Work out the finished part from the listing and answer in its coordinate system (mm). Face numbers are marked on the shaded views. A direction names the side the tool comes from. Give positions to 0.01 mm unless a question says otherwise; leave off trailing zeros. Loops run counter-clockwise (first coordinate to the right, second up) from the corner with the lowest first, then second, coordinate; pieces in that order, holes last. Notation, with made-up numbers: (86.5, 22) - (104.5, 22) arc R22 cw to (104.5, 36) - close; hole circle Ø1 at (61.25, -15.75). An arc over 180 degrees is marked (long way). One line per item, written item: value.
Autodesk Inventor part; units mm, degrees
ref_plane "Work Plane1" through (29, 0, 0) normal (0, -1, 0) x (1, 0, 0)
ref_plane "YZ Plane" through (0, 0, 0) normal (1, 0, 0) x (0, 1, 0)
ref_plane "XZ Plane" through (0, 0, 0) normal (0, 1, 0) x (-1, 0, 0)
sketch "Sketch1" plane through (0, 0, 0) normal (0, 0, 1) x (1, 0, 0)
  line L0 (-0.8667, 0) -> (5, 0)
  line L1 (5, 0) -> (5, 1.5)
  line L2 (5, 1.5) -> (1.25, 1.5)
  line L3 (1.25, 1.5) -> (0.9432, 1.5)
  line L4 (0.9432, 1.5) -> (0, 1.5)
  line L5 (0, 1.5) -> (0, 2.75)
  line L6 (0, 2.75) -> (-3, 2.75)
  line L7 (-3, 2.75) -> (-3, 1.4434)
  line L8 (-3, 1.4434) -> (-1.7, 1.4434)
  line L9 (-1.7, 1.4434) -> (-0.8667, 0)
  line L10 (-4.6, 0) -> (6.6, 0)
  line L11 (0, -0.55) -> (0, 3.3)
  line L12 (1.25, 1.5) -> (0, 1.5) construction
  dimension "d1" = 3.75
  dimension "d2" = 0.3068
  dimension "d3" = 3
  dimension "d4" = 1.3
  dimension "d5" = 60
  dimension "d6" = 3
  dimension "d7" = 3
  dimension "d8" = 2.8868
  dimension "d9" = 5.5
  dimension "d26" = 5
revolve "Body" add sketch "Sketch1" angle 360 about axis through (-0.8667, 0, 0) along (1, 0, 0)
sketch "Sketch2" plane through (-3, 0, 0) normal (-1, 0, 0) x (0, 0, 1)
  circle A0 centre (0, 0) radius 1.4434
  line L0 (0, -3.85) -> (0, 3.85)
  line L1 (-3.85, 0) -> (3.85, 0)
  line L2 (1.4434, 0) -> (0.7217, -1.25)
  line L3 (0.7217, -1.25) -> (-0.7217, -1.25)
  line L4 (-0.7217, -1.25) -> (-1.4434, 0)
  line L5 (-1.4434, 0) -> (-0.7217, 1.25)
  line L6 (-0.7217, 1.25) -> (0.7217, 1.25)
  line L7 (0.7217, 1.25) -> (1.4434, 0)
extrude "Slot" add sketch "Sketch2" against normal up to next contours L7 A0 | A0 L2 | L6 L0 A0 | A0 L0 L3 | L0 L6 A0 | A0 L3 L0 | L4 A0 | A0 L5
fillet "Fillet1" radius 0.3 1 edges at (-3, -2.75, 0)
thread "Thread"
chamfer "Chamfer1" distance 0.3067 distance2 0.3067 1 edges at (5, -1.5, 0) measured on face at (5, -0.2617, -0.7882)
ref_plane "Work Plane1" through (29, 0, 0) normal (0, -1, 0) x (1, 0, 0)
fillet "Fillet2" radius 0.1 1 edges at (0, -1.5, 0)
sketch "Sketch4" plane through (5, 0, 0) normal (1, 0, 0) x (0, 0, -1)
  circle A0 centre (0, 0) radius 2.75
  circle A1 centre (0, 0) radius 1.6
  point P0 (0, 0)
extrude "Extrusion3" cut sketch "Sketch4" against normal blind 1 contours A1
chamfer "Chamfer3" distance 0.5 angle 45 1 edges at (4, -1.5, 0)
equation "\"d1\" = GEL"
equation "\"d3\" = KOH"
equation "\"d4\" = INTI"
equation "\"d6\" = GD"
equation "\"d7\" = BDM"
equation "\"d8\" = 1.1547 * SW"
equation "\"d9\" = KOD"
equation "\"d26\" = NLG"
equation "\"d30\" = R"
equation "\"d17\" = RR"
equation "\"d13\" = GEL"
equation "\"d15\" = -0.5 * SPD + 0.5 * GD"
equation "\"d16\" = GUL"
equation "\"GD\" = 3"
equation "\"NLG\" = 5"
equation "\"GEL\" = 3.75"
equation "\"KOD\" = 5.5"
equation "\"KOH\" = 3"
equation "\"INTI\" = 1.3"
equation "\"GAL\" = 0.61345 * PTC"
equation "\"GUL\" = 0.61345 * PTC"
equation "\"BDM\" = NND"
equation "\"SW\" = 2.5"
equation "\"RR\" = 0.3"
equation "\"SPD\" = NND - 1.2269 * PTC"
equation "\"R\" = 0.1"
equation "\"TOA\" = 30deg"
equation "\"GD1\" = THREADDIA - 1.2269 * PTC"
equation "\"THREADDIA\" = 3"
equation "\"FAWI\" = 45deg"
equation "\"PTC\" = 0.5"
equation "\"NND\" = 3"
equation "\"E0\" = 1.155 * SW"
properties part number "ISO 4762 - M3 x 4" material "Stainless Steel, 440C"
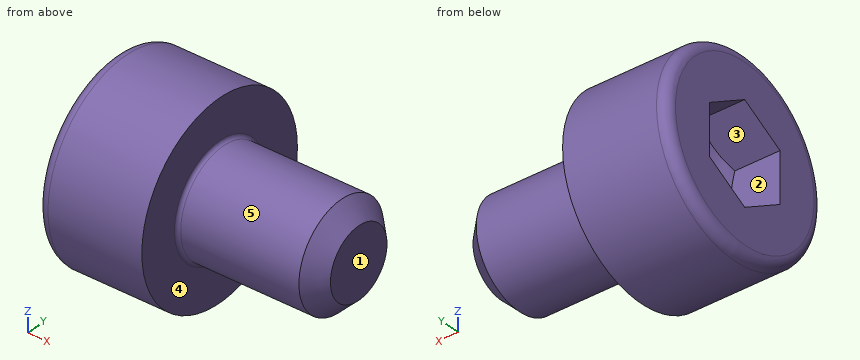
1. The mould has two halves that part along Y. Classify the marked faces 3, 4 and 5: released by +Y, released by -Y, zero draft, split by the parting line, or undercut.
Output:
face 3: undercut
face 4: zero draft
face 5: split by the parting line
2. For the marked faces 1 and 2, determine the directions among +Z, -Z, +X, -X, +Y, -Y from which every point of the face is accessible in a straight line to the end or side of a thin tool.
Output:
face 1: +Z, -Z, +X, +Y, -Y
face 2: -X
3. Section A-A (x = 1.75) is taken. Write down the section's boundary in (y, z), and give its area (3 significant figures).
Output:
outline: circle Ø3 at (0, 0)
area: 7.07 mm²
4. Section B-B (x = -0.5) is taken. Write down the section's boundary in (y, z), and give its area (3 significant figures).
Output:
outline: circle Ø5.5 at (0, 0)
area: 23.8 mm²
5. Flat-ended cylindrical pins translate along their axes: pin 1 Ø1.6 at (y, z) = (-1, -1) entering from +X; pin 2 Ø2 at (x, y) = (1.5, -0.5) entering from -Z; pin 3 Ø1 at (x, z) = (-0.5, -2) entering from +Y; pin 4 Ø1.5 at (x, y) = (1.5, -1.5) entering from +Z. Find the tip coordinate at first contact, or state that the pin passes through.
Output:
pin 1: stops at x = 4
pin 2: stops at z = -1.5
pin 3: stops at y = 2.3
pin 4: stops at z = 1.3
6. Find the intervals of material crossed by line 1 along X through (y, z) = (1.35, -1.4); line 2 along Z through (x, y) = (1, -0.4); line 3 along Z through (x, y) = (-2, 1), in increasing order.
Output:
line 1: x = -3 to 0
line 2: z = -1.45 to 1.45
line 3: z = -2.56 to -0.87, 0.87 to 2.56
